Design review of the part built by this model. Coordinates are the model's own, in mm. Face numbers are marked on the shaded views. A direction names the side the tool comes from. Coordinates: 2 decimals unless noted, no trailing zeros. Order: outer loops, then holes, each group sorted by start corner. A loop starts at its lowest first (then second) coordinate and runs counter-clockwise, first axis right, second up. Notation, with made-up numbers: M 89.5,60.25 L 142.5,60.25 A22 cw 142.5,88.25 Z; hole C 29,67 d7. An arc over 180 degrees is marked long. Answer as a JSON object with one key per item and string values.
from build123d import *

# Parameters (mm, degrees)
CROQUIS1_W              = 43
CROQUIS1_H              = 56.5
SALIENTE_EXTRUIR1_DEPTH = 9.53
CORTAR_EXTRUIR1_DEPTH   = 9.53
CORTAR_EXTRUIR2_REACH   = 38.758
CROQUIS3_R              = 2.75


with BuildPart() as part:
    # Croquis1 → Saliente-Extruir1 (new body)
    with BuildSketch(Plane.XY):
        Rectangle(CROQUIS1_W, CROQUIS1_H)
    extrude(amount=SALIENTE_EXTRUIR1_DEPTH)

    # Croquis2 → Cortar-Extruir1 (cut)
    with BuildSketch(Plane.XY.offset(9.53)):
        with BuildLine():
            ThreePointArc((-5.384, -15.485), (10.616, 0.515), (-5.384, 16.515))
            Line((-5.384, 16.515), (-21.5, 16.515))
            Line((-21.5, 16.515), (-21.5, -15.485))
            Line((-21.5, -15.485), (-5.384, -15.485))
        make_face()
    extrude(amount=-CORTAR_EXTRUIR1_DEPTH, mode=Mode.SUBTRACT)

    # Croquis3 → Cortar-Extruir2 (cut, up to next)
    with BuildSketch(Plane.XY.offset(9.53), mode=Mode.PRIVATE) as cortar_extruir2_sk1:
        with Locations((15.908, 0.383)):
            Circle(CROQUIS3_R)
    cortar_extruir2_tool1 = extrude(cortar_extruir2_sk1.sketch, amount=-CORTAR_EXTRUIR2_REACH, mode=Mode.PRIVATE) & part.part
    # Croquis3 → Cortar-Extruir2 (cut, up to next)
    with BuildSketch(Plane.XY.offset(9.53), mode=Mode.PRIVATE) as cortar_extruir2_sk2:
        with Locations((-5.542, 21.833)):
            Circle(CROQUIS3_R)
    cortar_extruir2_tool2 = extrude(cortar_extruir2_sk2.sketch, amount=-CORTAR_EXTRUIR2_REACH, mode=Mode.PRIVATE) & part.part
    # Croquis3 → Cortar-Extruir2 (cut, up to next)
    with BuildSketch(Plane.XY.offset(9.53), mode=Mode.PRIVATE) as cortar_extruir2_sk3:
        with Locations((-5.542, -21.105)):
            Circle(CROQUIS3_R)
    cortar_extruir2_tool3 = extrude(cortar_extruir2_sk3.sketch, amount=-CORTAR_EXTRUIR2_REACH, mode=Mode.PRIVATE) & part.part
    add(cortar_extruir2_tool1.solids().sort_by_distance((15.908, 0.383, 9.53))[0], mode=Mode.SUBTRACT)
    add(cortar_extruir2_tool2.solids().sort_by_distance((-5.542, 21.833, 9.53))[0], mode=Mode.SUBTRACT)
    add(cortar_extruir2_tool3.solids().sort_by_distance((-5.542, -21.105, 9.53))[0], mode=Mode.SUBTRACT)


solid = part.part
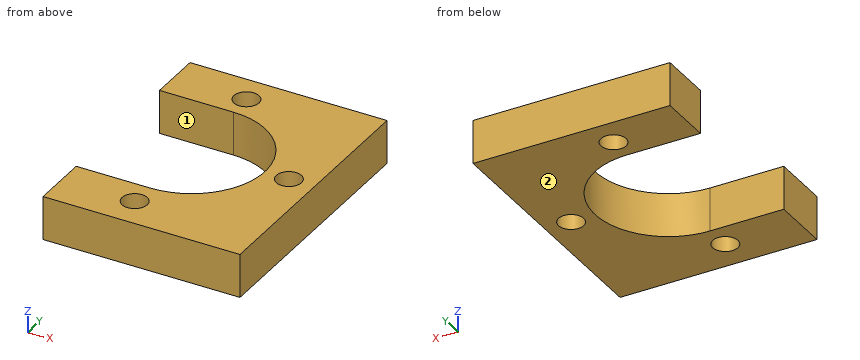
1) To check wall thickness, follow L1, parallel to X at y = -21, z = 2.25; L2, parallel to Y at x = -18.5, z = 3.25 (3 decimals); L3, parallel to Y at x = -0.5, z = 6.75. State the ranges of each line that lie inside material, in increasing order.
Taken from the geometry:
{"L1": "x = -21.5 to -8.29, -2.79 to 21.5", "L2": "y = -28.25 to -15.485, 16.515 to 28.25", "L3": "y = -28.25 to -14.72, 15.75 to 28.25"}
2) Add section A-A (x = -12.5). State the section outline as (y, z) points (3 decimals), and give its area (3 significant figures).
Taken from the geometry:
{"outline": "M -28.25,0 L -15.485,0 L -15.485,9.53 L -28.25,9.53 Z; M 16.515,0 L 28.25,0 L 28.25,9.53 L 16.515,9.53 Z", "area": "233 mm2"}
3) Add section D-D (x = -7.5). State the section outline as (y, z) points (3 decimals), and give its area (3 significant figures).
Taken from the geometry:
{"outline": "M -28.25,0 L -23.036,0 L -23.036,9.53 L -28.25,9.53 Z; M -19.174,0 L -15.485,0 L -15.485,9.53 L -19.174,9.53 Z; M 16.515,0 L 19.902,0 L 19.902,9.53 L 16.515,9.53 Z; M 23.764,0 L 28.25,0 L 28.25,9.53 L 23.764,9.53 Z", "area": "160 mm2"}
4) Tool access review of the marked faces 1 and 2: name each direction out of +Z, -Z, +X, -X, +Y, -Y from which nothing blocks a thin tool from reaching the whole face with its end or side.
Taken from the geometry:
{"face 1": "+Z, -Z, -X", "face 2": "-Z, +X, -X, +Y, -Y"}
5) Insertion check: pin 1 Ø4.5 at (x, y) = (-5.542, 21.833) entering from -Z. The pin has a flat end and moves straight along its axis. Give the tip position at first contact, or say it passes through.
Taken from the geometry:
{"pin 1": "passes through"}
6) Add section C-C (z = 3). State the section outline as (x, y) points (3 decimals).
Taken from the geometry:
{"outline": "M -21.5,-28.25 L 21.5,-28.25 L 21.5,28.25 L -21.5,28.25 L -21.5,16.515 L -5.384,16.515 A16 cw -5.384,-15.485 L -21.5,-15.485 Z; hole C -5.542,-21.105 d5.5; hole C -5.542,21.833 d5.5; hole C 15.908,0.383 d5.5"}
7) Add section B-B (y = 20.5). State the section outline as (x, z) points.
Taken from the geometry:
{"outline": "M -21.5,0 L -7.95,0 L -7.95,9.53 L -21.5,9.53 Z; M -3.14,0 L 21.5,0 L 21.5,9.53 L -3.14,9.53 Z"}
